Geometry check sheet. Reference: drawing and pictorial views, mm from the part's lowest x, y, z. A direction names the side the tool comes from. Coordinates: 2 decimals unless noted, no trailing zeros. Order: outer loops, then holes, each group sorted by start corner. A loop starts at its lowest first (then second) coordinate and runs counter-clockwise, first axis right, second up. Notation, with made-up numbers: (-12, -7) -> (15, -7) arc R16 cw to (15, 13) -> close; hole circle Ø3 at (-1, 57.5). An arc over 180 degrees is marked (long way). Use CSV: the item, a comma, the result in double quotes. Start each with the question number.
1) Tool access check on the marked faces 1, 2 and 3. Record the directions out of +Z, -Z, +X, -X, +Y, -Y that give a thin tool (end or side, any length) a straight path to the whole face; none if there is none.
2) Go/stop test with flat-tipped pins: pin 1 (16 mm diameter, centred on y = 94.5, z = 18.5, fed in from +X); pin 2 (6 mm diameter, centred on x = 37.5, z = 7, fed in from +Y). Record where each tip stops, or that it passes through.
3) Release check for a two-part mould opening along Z. For the marked faces 4, 5, 6 and 7 record: released by +Z, released by -Z, zero draft, split by the parting line, or undercut.
4) Sectioned sample at B-B on y = 107.5. Record the boundary of the cut face in (x, z).
5) Sectioned sample at A-A on z = 16. Record the boundary of the cut face in (x, y).
6) Scan lines: line 1 along Z through (x, y) = (6.25, 107.5); line 2 along X through (y, z) = (102, 5); line 3 along X through (y, z) = (5, 16). Record each from-to range of solid material in increasing order.
7) Sectioned sample at D-D on z = 24. Record the boundary of the cut face in (x, y).
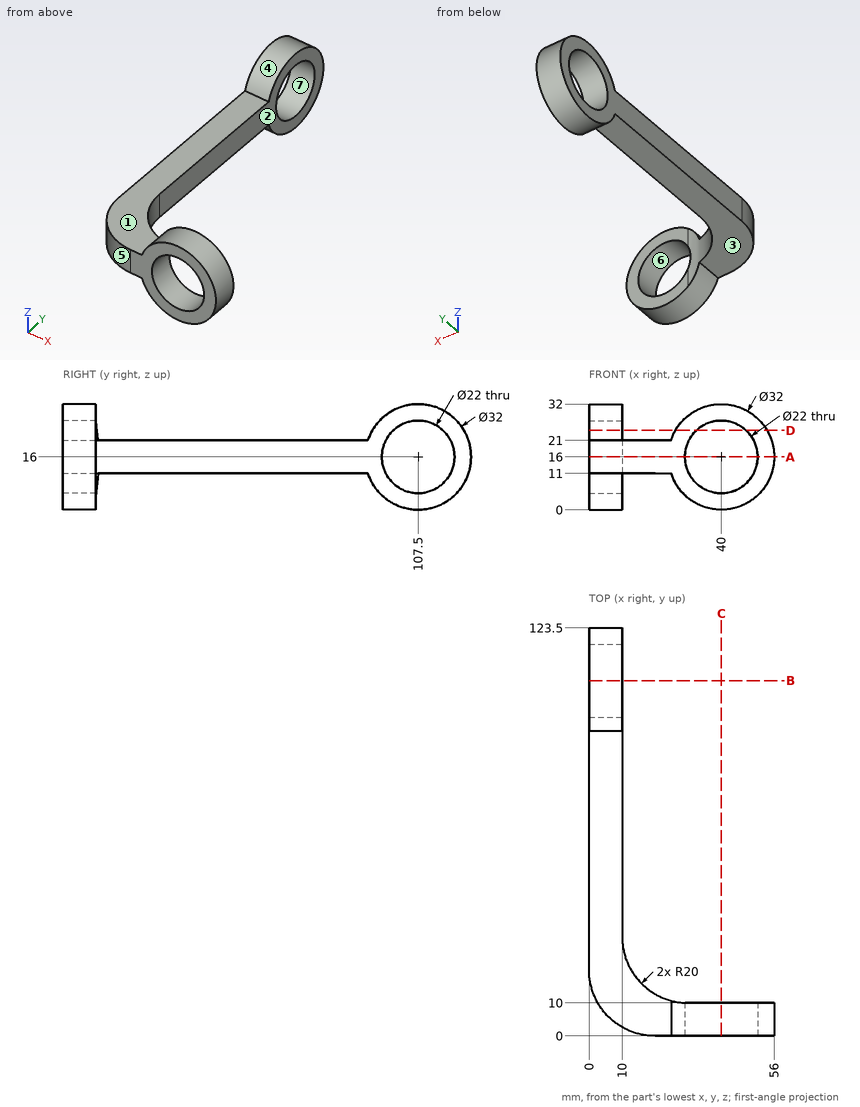
Answers follow:
1,face 1,"+Z, -X, -Y"
1,face 2,"+Z, -Z, +X, +Y"
1,face 3,"-Z, -X, -Y"
2,pin 1,"stops at x = 10"
2,pin 2,"stops at y = 10"
3,face 4,"split by the parting line"
3,face 5,"zero draft"
3,face 6,"undercut"
3,face 7,"undercut"
4,outline,"(0, 0) -> (10, 0) -> (10, 5) -> (0, 5) -> close; (0, 27) -> (10, 27) -> (10, 32) -> (0, 32) -> close"
5,outline,"(0, 20) arc R20 ccw to (20, 0) -> (29, 0) -> (29, 10.03) arc R20 cw to (10, 30) -> (10, 96.5) -> (0, 96.5) -> close; (0, 118.5) -> (10, 118.5) -> (10, 123.5) -> (0, 123.5) -> close; (51, 0) -> (56, 0) -> (56, 10) -> (51, 10) -> close"
6,line 1,"z = 0 to 5, 27 to 32"
6,line 2,"x = 0 to 10"
6,line 3,"x = 6.77 to 29, 51 to 56"
7,outline,"(0, 93.64) -> (10, 93.64) -> (10, 99.95) -> (0, 99.95) -> close; (0, 115.05) -> (10, 115.05) -> (10, 121.36) -> (0, 121.36) -> close; (26.14, 0) -> (32.45, 0) -> (32.45, 10) -> (30, 10) arc R20 cw to (26.14, 10.38) -> close; (47.55, 0) -> (53.86, 0) -> (53.86, 10) -> (47.55, 10) -> close"
